Autodesk Inventor part; units mm, degrees
ref_plane "Work Plane1" through (0, 0, 0) normal (0, 0, 1) x (1, 0, 0)
ref_plane "YZ Plane" through (0, 0, 0) normal (1, 0, 0) x (0, 1, 0)
ref_plane "XZ Plane" through (0, 0, 0) normal (0, 1, 0) x (-1, 0, 0)
ref_plane "Work Plane1" through (0, 0, 0) normal (0, 0, 1) x (1, 0, 0)
sketch "Sketch1" plane through (0, 0, 0) normal (0, 0, 1) x (1, 0, 0)
  line L0 (-75, -117.1) -> (75, -117.1)
  line L1 (75, -117.1) -> (75, 82.9)
  line L2 (75, 82.9) -> (-75, 82.9)
  line L3 (-75, 82.9) -> (-75, -117.1)
  point P0 (0, -17.1)
  dimension "d11" = 100
extrude "Extrusion1" add sketch "Sketch1" along normal blind 20
sketch "Sketch2" plane through (0, 0, 20) normal (0, 0, 1) x (1, 0, 0)
  circle A0 centre (0, -17.1) radius 15
  line L0 (75, 82.9) -> (-75, 82.9)
  line L1 (-75, 82.9) -> (-75, -117.1)
  circle A1 centre (-16.25, -0.85) radius 2.5
  circle A2 centre (16.25, -0.85) radius 2.5
  circle A3 centre (-16.25, -33.35) radius 2.5
  circle A4 centre (16.25, -33.35) radius 2.5
  point P0 (0, 0)
  dimension "d6" = 30
  dimension "d7" = 100
  dimension "d8" = 75
  dimension "d15" = 5
  dimension "d16" = 16.25
  dimension "d17" = 16.25
  dimension "d18" = 16.25
  dimension "d19" = 16.25
  dimension "d20" = 16.25
  dimension "d21" = 16.25
  dimension "d22" = 16.25
  dimension "d23" = 16.25
extrude "Extrusion2" cut sketch "Sketch2" against normal through all
sketch "Sketch4" plane through (0, 0, 0) normal (0, 0, -1) x (-1, 0, 0)
  circle A0 centre (0, -17.1) radius 15
  circle A1 centre (0, 52.9) radius 8
  circle A2 centre (0, -87.1) radius 8
  point P0 (0, 0)
  dimension "d33" = 70
  dimension "d34" = 70
  dimension "d35" = 16
extrude "Extrusion3" cut sketch "Sketch4" against normal blind 9 contours A1 | A2
sketch "Sketch5" plane through (0, 0, 20) normal (0, 0, 1) x (1, 0, 0)
  circle A0 centre (0, -17.1) radius 15
  point P0 (0, 0)
  point P1 (0, -87.1)
  point P2 (0, 52.9)
  dimension "d38" = 70
  dimension "d39" = 70
hole "Hole2" at (0, -87.1, 20) at (0, 52.9, 20) direction (0, 0, -1) diameter 6.647 end through all counterbore diameter 15 counterbore depth 5
equation "\"d17\" = d16"
equation "\"d18\" = d16"
equation "\"d19\" = d16"
equation "\"d20\" = d16"
equation "\"d21\" = d16"
equation "\"d22\" = d16"
equation "\"d23\" = d16"
properties part number "Soporte Pistón"
Verification items for the finished model (mm, model axes). A direction names the side the tool comes from. Coordinates: 2 decimals unless noted, no trailing zeros. Write each loop counter-clockwise with the first axis right and the second up, starting at its lowest first coordinate (ties: lowest second). Pieces come first, ordered by that corner, then holes. Notation, with made-up numbers: M -35.75,-32.5 L -17.75,-32.5 A35 cw -17.75,-0.5 Z; hole C 83.25,75.5 d8. An arc over 180 degrees is marked long. Answer as a JSON object with one key per item and string values. Group by question number.
(1) Tool access check on faces 4 (the face through (-0.33, 60.393, 17.465)), 5 (the face through (0, 49, 9)), 6 (the face through (13.752, -0.74, 10.14)). Record the directions out of +Z, -Z, +X, -X, +Y, -Y that give a thin tool (end or side, any length) a straight path to the whole face; none if there is none.
(2) Gauge pin test, flat ends, axial feed: pin 1 (13 mm diameter, centred on x = 0, y = -87.1, fed in from -Z); pin 2 (5.5 mm diameter, centred on x = 0, y = -87.1, fed in from +Z); pin 3 (4.5 mm diameter, centred on x = -2.5, y = -87, fed in from +Z). Record the tip position at first contact, or that the pin passes through.
(3) Cross-section at C-C, the plane z = 2.5. Record the cut outline in (x, y), and give its area (3 significant figures).
(4) Cross-section at A-A, the plane x = 0. State how many separate pieces and enclosed holes the cut face has, and give its area (3 significant figures).
(5) Material ranges on line 1 (Y direction, x = 16.25, z = 5.5); line 2 (Y direction, x = 0, z = 13.05); line 3 (X direction, y = -87.1, z = 19), recorded low to high.
(6) Release check for a two-part mould opening along Y. For faces 1 (the face through (1, 82.9, 10)), 2 (the face through (75, -18, 10)), 3 (the face through (-1, -90.27, 11.96)) record: +Y half, -Y half, draft (parallel to the pull), parting line (faces both ways), or undercut.
(7) Cross-section at B-B, the plane y = 52.9. Record the cut outline in (x, z), and give its area (3 significant figures).
(8) Cross-section at D-D, the plane y = -17.1. Record the cut outline in (x, z), and give its area (3 significant figures).
Reply:
{
 "1": {"face 4": "+Z", "face 5": "-Z", "face 6": "+Z, -Z"},
 "2": {"pin 1": "z = 9", "pin 2": "through", "pin 3": "z = 15"},
 "3": {"outline": "M -75,-117.1 L 75,-117.1 L 75,82.9 L -75,82.9 Z; hole C -16.25,-33.35 d5; hole C -16.25,-0.85 d5; hole C 0,-17.1 d30; hole C 0,-87.1 d16; hole C 0,52.9 d16; hole C 16.25,-33.35 d5; hole C 16.25,-0.85 d5", "area": "28,800 mm²"},
 "4": {"separate pieces": "4", "enclosed holes": "0", "area": "2,880 mm²"},
 "5": {"line 1": "-117.1 to -35.85, -30.85 to -3.35, 1.65 to 82.9", "line 2": "-117.1 to -90.42, -83.78 to -32.1, -2.1 to 49.58, 56.22 to 82.9", "line 3": "-75 to -7.5, 7.5 to 75"},
 "6": {"face 1": "+Y half", "face 2": "draft", "face 3": "undercut"},
 "7": {"outline": "M -75,0 L -8,0 L -8,9 L -3.32,9 L -3.32,15 L -7.5,15 L -7.5,20 L -75,20 Z; M 3.32,9 L 8,9 L 8,0 L 75,0 L 75,20 L 7.5,20 L 7.5,15 L 3.32,15 Z", "area": "2,740 mm²"},
 "8": {"outline": "M -75,0 L -15,0 L -15,20 L -75,20 Z; M 15,0 L 75,0 L 75,20 L 15,20 Z", "area": "2,400 mm²"}
}
